Geometry check sheet. Reference: the model listing, model coordinates, mm. A direction names the side the tool comes from. Round coordinates to 2 decimals unless told otherwise and drop trailing zeros. Write each loop counter-clockwise with the first axis right and the second up, starting at its lowest first coordinate (ties: lowest second). Pieces come first, ordered by that corner, then holes. Notation, with made-up numbers: M -19.75,8 L 11.25,8 A27 cw 11.25,46 Z; hole C -37.5,-0.75 d5. An arc over 180 degrees is marked long. Answer as CSV lines item,"result". Start each with the question number.
```python
from build123d import *

# Parameters (mm, degrees)
F1_DEPTH      = 50
F3_DEPTH      = 3
F5_DEPTH      = 6.5
F6_W          = 2
F6_H          = 22
F5_FACE1_W    = 6.5
F5_FACE1_H    = 22
F7_DEPTH      = 1.5
F8_W          = 2
F8_H          = 22
F9_DEPTH      = 1.5
F10_W         = 36
F10_H         = 22
F11_DEPTH     = 2
F12_W         = 20
F12_H         = 10
F13_DEPTH     = 28.4580883963
F14_T4_DEPTH  = 50
F14_T10_DEPTH = 50
F14_T16_DEPTH = 50
F14_T23_DEPTH = 50
F14_T29_DEPTH = 50
F15_R         = 5
F16_T4_DEPTH  = 7.0003952761
F17_R         = 2
F18_R         = 2
F19_R         = 7
F19_R_2       = 3
F20_DEPTH     = 1.5
F22_DEPTH     = 4.5
F24_DEPTH     = 4.5
F25_R         = 5
F26_R         = 5


# Not quite as in the source:
# - a fillet or chamfer that OpenCascade refuses, or shapes differently, is made with other operations: its cross-section is extruded or revolved along the edge and cut away or added


with BuildPart() as f1:
    # F0 (on Right) → F1 (new body)
    with BuildSketch(Plane.YZ):
        Polygon((-2, 0), (0, 0), (0, 2), (0, 24), (-2, 24), align=None)
        Polygon((0, 2), (0, 0), (11, 0), (16.274498548, 11.3111986384), (23.6785478522, 27.1892336111), (20.9596244911, 28.4570883963), (8.6224815594, 2), align=None)
        Polygon((16.274498548, 11.3111986384), (11, 0), (14.5032248927, 0), (19.1520257719, 9.9693856574), align=None)
    extrude(amount=F1_DEPTH)

    # F2 (on face) → F3 (cut, through all)
    with BuildSketch(Plane(origin=(0, 6.3164084922, -2.9453896519), x_dir=(1, 0, 0), z_dir=(0, -0.906307787, 0.4226182617))):
        with BuildLine():
            ThreePointArc((22, 23.4566337426), (25, 20.4566337426), (28, 23.4566337426))
            Line((28, 23.4566337426), (22, 23.4566337426))
        make_face()
        with BuildLine():
            Line((22, 23.4566337426), (28, 23.4566337426))
            ThreePointArc((28, 23.4566337426), (25, 26.4566337426), (22, 23.4566337426))
        make_face()
    extrude(amount=-F3_DEPTH, mode=Mode.SUBTRACT)

    # F4 (on face) → F5 (join)
    with BuildSketch(Plane.XZ.offset(2)):
        Polygon((2, 2), (2, 24), (0, 24), (0, 0), (50, 0), (50, 24), (48, 24), (48, 2), align=None)
    extrude(amount=F5_DEPTH)

    # F6 (on face) + F5_face1 (on face) → F7 (join)
    with BuildSketch(Plane.YZ.offset(2)):
        with Locations((-7.5, 13)):
            Rectangle(F6_W, F6_H)
    with BuildSketch(Plane(origin=(48, -5.25, 13), x_dir=(0, -1, 0), z_dir=(-1, 0, 0))):
        Rectangle(F5_FACE1_W, F5_FACE1_H)
    extrude(amount=F7_DEPTH, dir=(1, 0, 0))

    # F8 (on face) → F9 (join)
    with BuildSketch(Plane(origin=(48, 0, 0), x_dir=(0, -1, 0), z_dir=(-1, 0, 0))):
        with Locations((7.5, 13)):
            Rectangle(F8_W, F8_H)
    extrude(amount=F9_DEPTH)

    # F10 (on face) → F11 (cut)
    with BuildSketch(Plane.XZ.offset(2)):
        with Locations((25, 13)):
            Rectangle(F10_W, F10_H)
    extrude(amount=-F11_DEPTH, mode=Mode.SUBTRACT)

    # F12 (on Top) → F13 (cut, through all)
    with BuildSketch(Plane.XY):
        with Locations((25, 0.5)):
            Rectangle(F12_W, F12_H)
    extrude(amount=F13_DEPTH, mode=Mode.SUBTRACT)

    # F14: fillet of radius 5 on 1 edges, made by hand


with BuildPart() as f14_tool2:
    # F14_s3 → F14_t4 (new body)
    with BuildSketch(Plane.YZ):
        with BuildLine():
            ThreePointArc((9.9686691906, 4.8869086913), (8.1236282971, 2.7830427709), (5.4371302554, 2))
            Line((5.4371302554, 2), (8.6224815594, 2))
            Line((8.6224815594, 2), (9.9686691906, 4.8869086913))
        make_face()
    extrude(amount=F14_T4_DEPTH)

    split(bisect_by=Plane.XZ.offset(-5.5), keep=Keep.BOTTOM)

    split(bisect_by=Plane.YZ.offset(15), keep=Keep.BOTTOM)


with BuildPart() as f1_1:
    add(f1.part)

    # F14_t1: union F14_tool2
    add(f14_tool2.part)


with BuildPart() as f14_tool8:
    # F14_s9 → F14_t10 (new body)
    with BuildSketch(Plane.YZ):
        with BuildLine():
            ThreePointArc((9.9686691906, 4.8869086913), (8.1236282971, 2.7830427709), (5.4371302554, 2))
            Line((5.4371302554, 2), (8.6224815594, 2))
            Line((8.6224815594, 2), (9.9686691906, 4.8869086913))
        make_face()
    extrude(amount=F14_T10_DEPTH)

    split(bisect_by=Plane.XZ.offset(-5.5), keep=Keep.TOP)

    split(bisect_by=Plane.YZ.offset(15), keep=Keep.BOTTOM)


with BuildPart() as f1_2:
    add(f1_1.part)

    # F14_t7: union F14_tool8
    add(f14_tool8.part)


with BuildPart() as f14_tool14:
    # F14_s15 → F14_t16 (new body)
    with BuildSketch(Plane.YZ):
        with BuildLine():
            ThreePointArc((9.9686691906, 4.8869086913), (8.1236282971, 2.7830427709), (5.4371302554, 2))
            Line((5.4371302554, 2), (8.6224815594, 2))
            Line((8.6224815594, 2), (9.9686691906, 4.8869086913))
        make_face()
    extrude(amount=F14_T16_DEPTH)

    split(bisect_by=Plane.XZ.offset(-5.5), keep=Keep.BOTTOM)

    split(bisect_by=Plane.YZ.offset(15), keep=Keep.TOP)

    split(bisect_by=Plane.YZ.offset(35), keep=Keep.BOTTOM)


with BuildPart() as f1_3:
    add(f1_2.part)

    # F14_t13: union F14_tool14
    add(f14_tool14.part)


with BuildPart() as f14_tool21:
    # F14_s22 → F14_t23 (new body)
    with BuildSketch(Plane.YZ):
        with BuildLine():
            ThreePointArc((9.9686691906, 4.8869086913), (8.1236282971, 2.7830427709), (5.4371302554, 2))
            Line((5.4371302554, 2), (8.6224815594, 2))
            Line((8.6224815594, 2), (9.9686691906, 4.8869086913))
        make_face()
    extrude(amount=F14_T23_DEPTH)

    split(bisect_by=Plane.XZ.offset(-5.5), keep=Keep.BOTTOM)

    split(bisect_by=Plane.YZ.offset(35), keep=Keep.TOP)


with BuildPart() as f1_4:
    add(f1_3.part)

    # F14_t20: union F14_tool21
    add(f14_tool21.part)


with BuildPart() as f14_tool27:
    # F14_s28 → F14_t29 (new body)
    with BuildSketch(Plane.YZ):
        with BuildLine():
            ThreePointArc((9.9686691906, 4.8869086913), (8.1236282971, 2.7830427709), (5.4371302554, 2))
            Line((5.4371302554, 2), (8.6224815594, 2))
            Line((8.6224815594, 2), (9.9686691906, 4.8869086913))
        make_face()
    extrude(amount=F14_T29_DEPTH)

    split(bisect_by=Plane.XZ.offset(-5.5), keep=Keep.TOP)

    split(bisect_by=Plane.YZ.offset(35), keep=Keep.TOP)


with BuildPart() as f1_5:
    add(f1_4.part)

    # F14_t26: union F14_tool27
    add(f14_tool27.part)

    # F15
    f15_edges = [f1_5.edges().sort_by_distance(p)[0] for p in [
        (3.5, 0, 2),
        (46.5, 0, 2),
    ]]
    fillet(f15_edges, radius=F15_R)

    # F16: fillet of radius 2 on 1 edges, made by hand


with BuildPart() as f16_tool2:
    # F16_s3 → F16_t4 (new body)
    with BuildSketch(Plane.XY):
        with BuildLine():
            ThreePointArc((35, 3.5), (34.4142135624, 4.9142135624), (33, 5.5))
            Line((33, 5.5), (33, 5.54))
            Line((33, 5.54), (35.04, 5.54))
            Line((35.04, 5.54), (35.04, 3.5))
            Line((35.04, 3.5), (35, 3.5))
        make_face()
    extrude(amount=F16_T4_DEPTH)

    split(bisect_by=Plane.XY.offset(2), keep=Keep.BOTTOM)


with BuildPart() as f1_6:
    add(f1_5.part)

    # F16_t1: union F16_tool2
    add(f16_tool2.part)

    # F17#2 (call 1 of 2: OpenCascade refuses the feature's edges together)
    f17_2_edges = [f1_6.edges().sort_by_distance(p)[0] for p in [
        (15, -4.5, 1),
    ]]
    fillet(f17_2_edges, radius=F17_R)

    # F17 (call 2 of 2)
    f17_edges = [f1_6.edges().sort_by_distance(p)[0] for p in [
        (15, 5.5, 1.000198),
    ]]
    fillet(f17_edges, radius=F17_R)

    # F18
    f18_edges = [f1_6.edges().sort_by_distance(p)[0] for p in [
        (35, -4.5, 1),
    ]]
    fillet(f18_edges, radius=F18_R)

    # F19 (on face) → F20 (cut)
    with BuildSketch(Plane(origin=(0, 6.3164084922, -2.9453896519), x_dir=(1, 0, 0), z_dir=(0, -0.906307787, 0.4226182617))):
        with Locations((25, 23.4566337426)):
            Circle(F19_R)
        with Locations((25, 23.4566337426)):
            Circle(F19_R_2, mode=Mode.SUBTRACT)
    extrude(amount=-F20_DEPTH, mode=Mode.SUBTRACT)

    # F21 (on face) → F22 (join, through all)
    with BuildSketch(Plane.XZ.offset(2)):
        Polygon((48, 23), (48, 24), (47.5, 23), align=None)
    extrude(amount=F22_DEPTH)

    # F23 (on face) → F24 (join, through all)
    with BuildSketch(Plane.XZ.offset(2)):
        Polygon((2.5, 23), (2, 24), (2, 23), align=None)
    extrude(amount=F24_DEPTH)

    # F25
    f25_edges = [f1_6.edges().sort_by_distance(p)[0] for p in [
        (50, 22.319086, 27.823161),
        (0, 22.319086, 27.823161),
    ]]
    fillet(f25_edges, radius=F25_R)

    # F26
    f26_edges = [f1_6.edges().sort_by_distance(p)[0] for p in [
        (7, -1, 24),
        (43, -1, 24),
    ]]
    fillet(f26_edges, radius=F26_R)


solid = f1_6.part
```
1) Section check A-A, the plane x = 30. Record the cut outline in (y, z), plus the area to 3 significant figures.
2) Access from +Z, -Z, +X, -X, +Y, -Y to the whole of each face (thin tool, end or side, straight path). Record for faces 4 (the cylindrical face through (15.57, 4.9, 0.99)), 5 (the flat face through (2.254, -4.219, 23.493)), 6 (the flat face through (43, -1, 10)).
3) Section check C-C, the plane z = 6.25. Record the cut outline in (x, y).
4) Section check B-B, the plane y = -5.5. Record the cut outline in (x, z), plus the area to 4 significant figures.
5) Section check D-D, the plane x = 23.5. Record the cut outline in (y, z), plus the area to 3 significant figures.
6) Mould release check, pull along Y, two halves, no side actions. Record for faces 1 (the flat face through (24.65, 20.747, 20.903)), 2 (the flat face through (24.7, 13.1, 11.6)), 3 (the flat face through (50, -0.4, 12.2)): released by +Y, released by -Y, zero draft, split by the parting line, or undercut.
7) Go/stop test with flat-tipped pins: pin 1 (5.5 mm diameter, centred on x = 3.5, z = 17, fed in from +Y); pin 2 (8 mm diameter, centred on x = 36, z = 5.5, fed in from -Y); pin 3 (6 mm diameter, centred on x = 9.5, z = 19.5, fed in from +Y); pin 4 (2.5 mm diameter, centred on x = 44.5, z = 15, fed in from -Y). Record where each tip stops, or that it passes through.
8) Scan lines: line 1 (X direction, y = -4.5, z = 14.75); line 2 (Z direction, x = 11.5, y = -4); line 3 (Y direction, x = 5, z = 7.25). Record each from-to range of solid material in increasing order. Write a range as from..to.
Results:
1,outline,"M -8.5,0 L -4.5,0 L -4.5,2 L -8.5,2 Z; M 5.5,0 L 14.5,0 L 19.15,9.97 L 16.27,11.31 L 23.68,27.19 L 20.96,28.46 L 18.3,22.75 L 19.66,22.12 L 15.52,13.24 L 14.16,13.87 L 9.97,4.89 A5 cw 5.5,2 Z"
1,area,"130 mm^2"
2,face 4,"+Z, -Z"
2,face 5,"+Z"
2,face 6,"+Z, -Y"
3,outline,"M 0,-8.5 L 3.5,-8.5 L 3.5,-6.5 L 2,-6.5 L 2,-2 L 7,-2 L 7,0.06 L 0,0.06 Z; M 0,10.6 L 50,10.6 L 50,17.42 L 0,17.42 Z; M 43,-2 L 48,-2 L 48,-6.5 L 46.5,-6.5 L 46.5,-8.5 L 50,-8.5 L 50,0.06 L 43,0.06 Z"
4,outline,"M 0,0 L 50,0 L 50,24 L 48,24 L 47.5,23 L 48,23 L 48,2 L 2,2 L 2,23 L 2.5,23 L 2,24 L 0,24 Z"
4,area,"188.5 mm^2"
5,outline,"M -8.5,0 L -4.5,0 L -4.5,2 L -8.5,2 Z; M 5.5,0 L 14.5,0 L 19.15,9.97 L 16.27,11.31 L 17.85,14.69 L 16.49,15.32 L 14.7,11.48 L 13.34,12.12 L 9.97,4.89 A5 cw 5.5,2 Z; M 18.69,20.03 L 20.05,19.4 L 23.68,27.19 L 20.96,28.46 L 19.12,24.51 L 20.48,23.88 Z"
5,area,"116 mm^2"
6,face 1,"released by +Y"
6,face 2,"undercut"
6,face 3,"zero draft"
7,pin 1,"stops at y = 20.21"
7,pin 2,"stops at y = -8.5"
7,pin 3,"stops at y = 21.49"
7,pin 4,"stops at y = -2"
8,line 1,"x = 0..2, 48..50"
8,line 2,"z = 0..2"
8,line 3,"y = -2..0, 11.07..17.88"
